Check sheet for the modelled part. Datum: model origin and axes. Units: mm. A direction names the side the tool comes from. Give positions to 0.01 mm unless a question says otherwise; leave off trailing zeros. Write each loop counter-clockwise with the first axis right and the second up, starting at its lowest first coordinate (ties: lowest second). Pieces come first, ordered by that corner, then holes. Notation, with made-up numbers: (44.5, 38) -> (98.5, 38) arc R13 ccw to (98.5, 51) -> close; hole circle Ø7 at (9, 44). An arc over 180 degrees is marked (long way). Answer as a JSON object with one key per item and string values.
from build123d import *

# Parameters (mm, degrees)
SKETCH1_R                     = 10
BOSS_EXTRUDE1_DEPTH           = 26
BOSS_EXTRUDE1_TAPER           = 2
BOSS_EXTRUDE1_OTHER_WAY_DEPTH = 6
BOSS_EXTRUDE1_OTHER_WAY_TAPER = -2
CUT_EXTRUDE1_DEPTH            = 30.740019936
CUT_EXTRUDE1_DEPTH_BACK       = 30.740019936
SKETCH3_W                     = 10
SKETCH3_H                     = 6
CUT_EXTRUDE2_DEPTH            = 25
CUT_EXTRUDE3_DEPTH            = 32.805094434
CUT_EXTRUDE3_DEPTH_BACK       = 32.805094434
SKETCH4_R                     = 1.5
FILLET2_SIZE                  = 5
CUT_EXTRUDE5_DEPTH            = 30.740020092
CUT_EXTRUDE5_DEPTH_BACK       = 30.740020092
SKETCH8_W                     = 10
SKETCH8_H                     = 6
CUT_EXTRUDE6_DEPTH            = 31.050909814
CUT_EXTRUDE7_DEPTH            = 30.668744533
CUT_EXTRUDE8_DEPTH            = 32.738456946
CUT_EXTRUDE8_DEPTH_BACK       = 32.738456946
SKETCH9_R                     = 1.351518808
FILLET3_SIZE                  = 5


with BuildPart() as part:
    # Sketch1 → Boss-Extrude1 (new body)
    with BuildSketch(Plane(origin=(0, 0, 0), x_dir=(1, 0, 0), z_dir=(0, 1, 0))):
        Circle(SKETCH1_R)
    extrude(amount=BOSS_EXTRUDE1_DEPTH, taper=BOSS_EXTRUDE1_TAPER)

    # Sketch1 → Boss-Extrude1 other way (add)
    with BuildSketch(Plane(origin=(0, 0, 0), x_dir=(1, 0, 0), z_dir=(0, 1, 0))):
        Circle(SKETCH1_R)
    extrude(amount=-BOSS_EXTRUDE1_OTHER_WAY_DEPTH, taper=BOSS_EXTRUDE1_OTHER_WAY_TAPER)

    # Sketch2 → Cut-Extrude1 (cut, two sides: drawn at the far end of the back side and taken through both)
    with BuildSketch(Plane(origin=(0, 0, 0), x_dir=(0, 0, -1), z_dir=(1, 0, 0)).offset(-CUT_EXTRUDE1_DEPTH_BACK)):
        Polygon((-0.907940007, 26), (-0.907940007, 20), (-13.415596948, 7.492343059), (-13.415596948, 26), align=None)
    extrude(amount=CUT_EXTRUDE1_DEPTH + CUT_EXTRUDE1_DEPTH_BACK, mode=Mode.SUBTRACT)

    # Sketch3 → Cut-Extrude2 (cut)
    with BuildSketch(Plane.XY.offset(0.907940007)):
        with Locations((0, 23)):
            Rectangle(SKETCH3_W, SKETCH3_H)
    extrude(amount=-CUT_EXTRUDE2_DEPTH, mode=Mode.SUBTRACT)

    # Sketch4 → Cut-Extrude3 (cut, two sides: drawn at the far end of the back side and taken through both)
    with BuildSketch(Plane(origin=(-5, 0, 0), x_dir=(0, 0, -1), z_dir=(1, 0, 0)).offset(-CUT_EXTRUDE3_DEPTH_BACK)):
        with Locations((1.592059993, 23.5)):
            Circle(SKETCH4_R)
    extrude(amount=CUT_EXTRUDE3_DEPTH + CUT_EXTRUDE3_DEPTH_BACK, mode=Mode.SUBTRACT)

    # Fillet2
    # a fillet whose section is not a circle: 5 mm, written as the material it takes off along each edge
    with BuildSketch(Plane(origin=(-7.5, 26, 0.907940007), x_dir=(0, -1, 0), z_dir=(1, 0, 0))) as fillet2_piece_1:
        with BuildLine():
            Bezier((FILLET2_SIZE, 0), (0, 0), (0, FILLET2_SIZE), weights=[1, 1.5, 1])
            Line((0, FILLET2_SIZE), (0, 0))
            Line((0, 0), (FILLET2_SIZE, 0))
        make_face()
    extrude(amount=29.046612618, mode=Mode.SUBTRACT)
    with BuildSketch(Plane(origin=(-21.546612618, 26, 0.907940007), x_dir=(0, 0, -1), z_dir=(1, 0, 0))) as fillet2_piece_2:
        with BuildLine():
            Bezier((FILLET2_SIZE, 0), (0, 0), (0, -FILLET2_SIZE), weights=[1, 1.5, 1])
            Line((0, -FILLET2_SIZE), (0, 0))
            Line((0, 0), (FILLET2_SIZE, 0))
        make_face()
    extrude(amount=29.046612618, mode=Mode.SUBTRACT)

    # Sketch7 → Cut-Extrude5 (cut, two sides: drawn at the far end of the back side and taken through both)
    with BuildSketch(Plane(origin=(0, 0, 0), x_dir=(0, 0, -1), z_dir=(1, 0, 0)).offset(-CUT_EXTRUDE5_DEPTH_BACK)):
        Polygon((-0.873019237, -6), (-0.873019237, 0), (-11.31781305, 10.444793812), (-11.31781305, -6), align=None)
    extrude(amount=CUT_EXTRUDE5_DEPTH + CUT_EXTRUDE5_DEPTH_BACK, mode=Mode.SUBTRACT)

    # Sketch8 → Cut-Extrude6 (cut, through all)
    with BuildSketch(Plane.XY.offset(0.873019237)):
        with Locations((0, -3)):
            Rectangle(SKETCH8_W, SKETCH8_H)
    extrude(amount=-CUT_EXTRUDE6_DEPTH, mode=Mode.SUBTRACT)

    # Sketch6 → Cut-Extrude7 (cut, through all)
    with BuildSketch(Plane(origin=(0, 20, 0), x_dir=(1, 0, 0), z_dir=(0, 1, 0))):
        with BuildLine():
            Line((5, 5.321009098), (5, -0.907940007))
            Line((5, -0.907940007), (-5, -0.907940007))
            Line((-5, -0.907940007), (-5, 5.321009098))
            ThreePointArc((-5, 5.321009098), (0, 7.30158461), (5, 5.321009098))
        make_face()
    extrude(amount=-CUT_EXTRUDE7_DEPTH, mode=Mode.SUBTRACT)

    # Sketch9 → Cut-Extrude8 (cut, two sides: drawn at the far end of the back side and taken through both)
    with BuildSketch(Plane(origin=(-5, 0, 0), x_dir=(0, 0, -1), z_dir=(1, 0, 0)).offset(-CUT_EXTRUDE8_DEPTH_BACK)):
        with Locations((1.626980763, -3.5)):
            Circle(SKETCH9_R)
    extrude(amount=CUT_EXTRUDE8_DEPTH + CUT_EXTRUDE8_DEPTH_BACK, mode=Mode.SUBTRACT)

    # Fillet3
    # a fillet whose section is not a circle: 5 mm, written as the material it takes off along each edge
    with BuildSketch(Plane(origin=(22.672130078, -6, 0.873019237), x_dir=(0, 0, -1), z_dir=(-1, 0, 0))) as fillet3_piece_1:
        with BuildLine():
            Bezier((FILLET3_SIZE, 0), (0, 0), (0, -FILLET3_SIZE), weights=[1, 1, 1])
            Line((0, -FILLET3_SIZE), (0, 0))
            Line((0, 0), (FILLET3_SIZE, 0))
        make_face()
    extrude(amount=30.172130078, mode=Mode.SUBTRACT)
    with BuildSketch(Plane(origin=(7.5, -6, 0.873019237), x_dir=(0, 1, 0), z_dir=(-1, 0, 0))) as fillet3_piece_2:
        with BuildLine():
            Bezier((FILLET3_SIZE, 0), (0, 0), (0, FILLET3_SIZE), weights=[1, 1, 1])
            Line((0, FILLET3_SIZE), (0, 0))
            Line((0, 0), (FILLET3_SIZE, 0))
        make_face()
    extrude(amount=30.172130078, mode=Mode.SUBTRACT)


solid = part.part
1. Sectioned sample at C-C, the plane y = 10.5. Enter the section's corners in (x, z), plus the area to 3 significant figures.
Determined:
{"outline": "circle Ø19.27 at (0, 0); hole (-5, -5.32) arc R7.3 ccw to (5, -5.32) -> (5, 0.91) -> (-5, 0.91) -> close", "area": "216 mm^2"}
2. Sectioned sample at B-B, the plane y = 20.5. Enter the section's corners in (x, z), plus the area to 3 significant figures.
Determined:
{"outline": "(-9.24, 0.91) arc R9.28 ccw to (-5, -7.82) -> (-5, 0.91) -> close; (5, -7.82) arc R9.28 ccw to (9.24, 0.91) -> (5, 0.91) -> close", "area": "55.0 mm^2"}
3. Scan lines: L1, parallel to X at y = 11.5, z = -2.25; L2, parallel to Y at x = 6.25, z = -2.75; L3, parallel to Z at x = 0.25, y = 14.5. Record each from-to range of solid material in increasing order. Write a range as [from, to].
Determined:
{"L1": "[-9.33, -5], [5, 9.33]", "L2": "[-5.89, -4.25], [-2.75, 22.55], [24.45, 25.95]", "L3": "[-9.49, -7.3], [0.91, 6.41]"}
4. Sectioned sample at A-A, the plane x = 0. Enter the section's corners in (y, z).
Determined:
{"outline": "(0, -10) -> (20, -9.3) -> (20, -7.3) -> (0, -7.3) -> close; (0.03, 0.91) -> (20, 0.91) -> (11.3, 9.61) -> (8.82, 9.69) -> close"}
5. Mould release check, pull along Y, two halves, no side actions. Record for faces 5 (the face through (-7.2, 20.5, 0.908)), 6 (the face through (7, -6, -6)), 7 (the face through (-6, 26, -5)), 8 (the face through (-7.604, -3.441, -0.277)): released by +Y, released by -Y, zero draft, split by the parting line, or undercut.
Determined:
{"face 5": "zero draft", "face 6": "released by -Y", "face 7": "released by +Y", "face 8": "undercut"}
6. Access from +Z, -Z, +X, -X, +Y, -Y to the whole of each face (thin tool, end or side, straight path). Record for faces 1 (the face through (7.1, 20.5, 0.908)), 2 (the face through (0, 20, -8)), 3 (the face through (0, 10, 0.908)), 4 (the face through (7.5, -0.5, 0.873)).
Determined:
{"face 1": "+Z, +X, -X, +Y", "face 2": "+Z, -Z, +Y", "face 3": "+Y, -Y", "face 4": "+Z, +X, -X, -Y"}
7. Sectioned sample at D-D, the plane y = -3. State how many separate pieces and enclosed holes the cut face has, plus the area to 3 significant figures.
Determined:
{"separate pieces": "4", "enclosed holes": "0", "area": "45.1 mm^2"}
8. Go/stop test with flat-tipped pins: P1, Ø2, axis at x = -1.5, z = -7, coming from the +Y side; P2, Ø8, axis at x = 7.5, y = 19.5, coming from the +Z side; P3, Ø0.5, axis at x = 7.5, y = -0.5, coming from the +Z side. Record where each tip stops, or that it passes through.
Determined:
{"P1": "y = 20", "P2": "z = 5.41", "P3": "z = 0.87"}
